The listing builds one solid part. Answer for the finished solid, in the listing's coordinates (mm). Face numbers are marked on the shaded views. A direction names the side the tool comes from. Coordinates: 2 decimals unless noted, no trailing zeros. Order: outer loops, then holes, each group sorted by start corner. A loop starts at its lowest first (then second) coordinate and runs counter-clockwise, first axis right, second up.
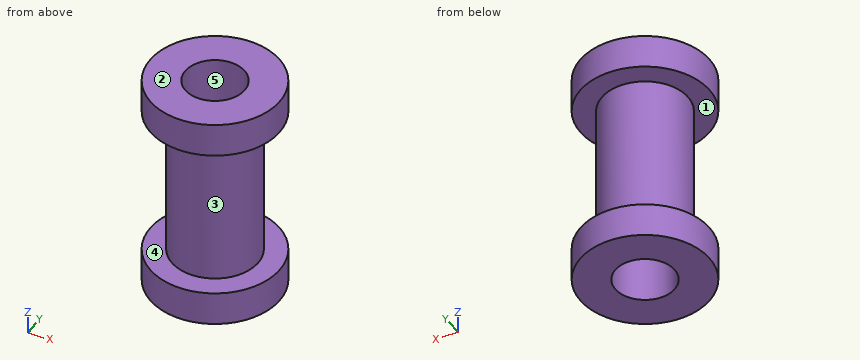
```python
from build123d import *

# Parameters (mm, degrees)
SKETCH1_R           = 25.4
SKETCH1_R_2         = 17.5
BOSS_EXTRUDE1_DEPTH = 65
BOSS_EXTRUDE2_START = -20
SKETCH2_R           = 38.1
SKETCH2_R_2         = 25.4
BOSS_EXTRUDE2_DEPTH = 20


with BuildPart() as part:
    # Sketch1 → Boss-Extrude1 (new, symmetric)
    with BuildSketch(Plane.XY):
        Circle(SKETCH1_R)
        Circle(SKETCH1_R_2, mode=Mode.SUBTRACT)
    extrude(amount=BOSS_EXTRUDE1_DEPTH, both=True)

    # Sketch2 → Boss-Extrude2 (add)
    with BuildSketch(Plane(origin=(0, 0, -65), x_dir=(-1, 0, 0), z_dir=(0, 0, -1)).offset(BOSS_EXTRUDE2_START)):
        Circle(SKETCH2_R)
        Circle(SKETCH2_R_2, mode=Mode.SUBTRACT)
    boss_extrude2 = extrude(amount=BOSS_EXTRUDE2_DEPTH)

    # Mirror1: Boss-Extrude2 across plane
    add(boss_extrude2.mirror(Plane.XY))


solid = part.part
```
1) Straight lines are drawn through the part: probe 1 along Z at (x, y) = (26.5, 3.5); probe 2 along X at (y, z) = (1, -36); probe 3 along Y at (x, z) = (0, -16). For each, find the intervals that lie inside material, in ascending order.
2) Each of these flat-tipped pins is pushed along its axis until it touches: P1, Ø12, axis at x = 14, z = -46, coming from the +Y side; P2, Ø6, axis at x = 28.5, z = 31, coming from the +Y side; P3, Ø4, axis at x = 21, z = 12, coming from the -Y side; P4, Ø12, axis at y = 14, z = 50, coming from the -X side. Where does it stop, or does it pass through?
3) For the marked faces 1 and 2, determine the directions among +Z, -Z, +X, -X, +Y, -Y from which every point of the face is accessible in a straight line to the end or side of a thin tool.
4) A cutting plane is placed at C-C, the plane z = 56. Write down the section's boundary in (x, y), plus the area to 3 significant figures.
5) A cutting plane is placed at A-A, the plane y = 0. Write down the section's boundary in (x, z).
6) A cutting plane is placed at D-D, the plane x = -20.5. Write down the section's boundary in (y, z).
7) The mould has two halves that part along X. Classify the marked faces 3, 4 and 5: released by +X, released by -X, zero draft, split by the parting line, or undercut.
Working result:
1. probe 1: z = -65 to -45, 45 to 65
1. probe 2: x = -25.38 to -17.47, 17.47 to 25.38
1. probe 3: y = -25.4 to -17.5, 17.5 to 25.4
2. P1: stops at y = 37.25
2. P2: passes through
2. P3: stops at y = -16.86
2. P4: stops at x = -37.25
3. face 1: none
3. face 2: +Z, +X, -X, +Y, -Y
4. outline: circle Ø76.2 at (0, 0); hole circle Ø35 at (0, 0)
4. area: 3,600 mm2
5. outline: (-38.1, -65) - (-17.5, -65) - (-17.5, 65) - (-38.1, 65) - (-38.1, 45) - (-25.4, 45) - (-25.4, -45) - (-38.1, -45) - close; (17.5, -65) - (38.1, -65) - (38.1, -45) - (25.4, -45) - (25.4, 45) - (38.1, 45) - (38.1, 65) - (17.5, 65) - close
6. outline: (-32.11, -65) - (32.11, -65) - (32.11, -45) - (15, -45) - (15, 45) - (32.11, 45) - (32.11, 65) - (-32.11, 65) - (-32.11, 45) - (-15, 45) - (-15, -45) - (-32.11, -45) - close
7. face 3: split by the parting line
7. face 4: zero draft
7. face 5: undercut
